from build123d import *

# Parameters (mm, degrees)
SKETCH1_W           = 80
SKETCH1_H           = 65
BOSS_EXTRUDE1_DEPTH = 10
SKETCH2_W           = 75
SKETCH2_H           = 60
CUT_EXTRUDE1_DEPTH  = 8
FILLET4_R           = 2
FILLET5_R           = 3
SKETCH3_W           = 80
SKETCH3_H           = 65
SKETCH3_W_2         = 77
SKETCH3_H_2         = 62
CUT_EXTRUDE2_DEPTH  = 1.5
FILLET7_R           = 4
SKETCH4_R           = 1.27
BOSS_EXTRUDE2_DEPTH = 3
SKETCH5_W           = 6
SKETCH5_H           = 3.5
CUT_EXTRUDE3_DEPTH  = 102.642756751
FILLET8_R           = 0.5
SKETCH8_W           = 69
SKETCH8_H           = 3
CUT_EXTRUDE4_DEPTH  = 1.5
SKETCH9_W           = 69
SKETCH9_H           = 3
CUT_EXTRUDE5_DEPTH  = 1.5


with BuildPart() as part:
    # Sketch1 → Boss-Extrude1 (new body)
    with BuildSketch(Plane(origin=(0, 0, 0), x_dir=(1, 0, 0), z_dir=(0, 1, 0))):
        with Locations((40, 32.5)):
            Rectangle(SKETCH1_W, SKETCH1_H)
    extrude(amount=BOSS_EXTRUDE1_DEPTH)

    # Sketch2 → Cut-Extrude1 (cut)
    with BuildSketch(Plane(origin=(0, 10, 0), x_dir=(1, 0, 0), z_dir=(0, 1, 0))):
        with Locations((40, 32.5)):
            Rectangle(SKETCH2_W, SKETCH2_H)
    extrude(amount=-CUT_EXTRUDE1_DEPTH, mode=Mode.SUBTRACT)

    # Fillet4
    fillet4_edges = [part.edges().sort_by_distance(p)[0] for p in [
        (40, 0, -65),
        (80, 0, -32.5),
        (40, 0, 0),
        (0, 0, -32.5),
    ]]
    fillet(fillet4_edges, radius=FILLET4_R)

    # Fillet5
    # the kernel refuses this fillet: 3 mm, written as the material it adds along each edge
    with BuildSketch(Plane(origin=(2.5, 10, -2.5), x_dir=(0, 0, -1), z_dir=(0, -1, 0)), Plane(origin=(77.5, 10, -62.5), x_dir=(0, 0, 1), z_dir=(0, -1, 0)), Plane(origin=(77.5, 10, -2.5), x_dir=(-1, 0, 0), z_dir=(0, -1, 0))) as fillet5_piece_1:
        with BuildLine():
            CenterArc((FILLET5_R, FILLET5_R), FILLET5_R, 180, 90)
            Line((0, FILLET5_R), (0, 0))
            Line((0, 0), (FILLET5_R, 0))
        make_face()
    extrude(amount=8)
    with BuildSketch(Plane(origin=(2.5, 10, -62.5), x_dir=(0, 0, 1), z_dir=(0, -1, 0))) as fillet5_piece_2:
        with BuildLine():
            CenterArc((FILLET5_R, -FILLET5_R), FILLET5_R, 90, 90)
            Line((0, -FILLET5_R), (0, 0))
            Line((0, 0), (FILLET5_R, 0))
        make_face()
    extrude(amount=8)
    # the kernel refuses this fillet: 3 mm, written as the material it takes off along each edge
    with BuildSketch(Plane(origin=(77, 0, -62), x_dir=(0, 0, -1), z_dir=(-1, 0, 0))) as fillet5_2_piece_1:
        with BuildLine():
            CenterArc((1, -2), 2, 0, 90)
            Line((3, -2), (3, 0))
            Line((3, 0), (1, 0))
        make_face()
    revolve(axis=Axis((77, 0, -62), (0, -1, 0)), revolution_arc=90, mode=Mode.SUBTRACT)
    with BuildSketch(Plane(origin=(77, 0, -3), x_dir=(1, 0, 0), z_dir=(0, 0, -1))) as fillet5_2_piece_2:
        with BuildLine():
            CenterArc((1, -2), 2, 0, 90)
            Line((3, -2), (3, 0))
            Line((3, 0), (1, 0))
        make_face()
    revolve(axis=Axis((77, 0, -3), (0, -1, 0)), revolution_arc=90, mode=Mode.SUBTRACT)
    with BuildSketch(Plane(origin=(3, 0, -62), x_dir=(-1, 0, 0), z_dir=(0, 0, 1))) as fillet5_2_piece_3:
        with BuildLine():
            CenterArc((1, -2), 2, 0, 90)
            Line((3, -2), (3, 0))
            Line((3, 0), (1, 0))
        make_face()
    revolve(axis=Axis((3, 0, -62), (0, -1, 0)), revolution_arc=90, mode=Mode.SUBTRACT)
    with BuildSketch(Plane(origin=(3, 0, -3), x_dir=(0, 0, 1), z_dir=(1, 0, 0))) as fillet5_2_piece_4:
        with BuildLine():
            CenterArc((1, -2), 2, 0, 90)
            Line((3, -2), (3, 0))
            Line((3, 0), (1, 0))
        make_face()
    revolve(axis=Axis((3, 0, -3), (0, -1, 0)), revolution_arc=90, mode=Mode.SUBTRACT)
    with BuildSketch(Plane(origin=(0, 0, -65), x_dir=(0, 0, 1), z_dir=(0, 1, 0)), Plane(origin=(0, 0, 0), x_dir=(1, 0, 0), z_dir=(0, 1, 0))) as fillet5_2_piece_5:
        with BuildLine():
            CenterArc((FILLET5_R, FILLET5_R), FILLET5_R, 180, 90)
            Line((0, FILLET5_R), (0, 0))
            Line((0, 0), (FILLET5_R, 0))
        make_face()
    extrude(amount=17.5, mode=Mode.SUBTRACT)
    with BuildSketch(Plane(origin=(80, 0, -65), x_dir=(0, 0, 1), z_dir=(0, 1, 0)), Plane(origin=(80, 0, 0), x_dir=(-1, 0, 0), z_dir=(0, 1, 0))) as fillet5_2_piece_6:
        with BuildLine():
            CenterArc((FILLET5_R, -FILLET5_R), FILLET5_R, 90, 90)
            Line((0, -FILLET5_R), (0, 0))
            Line((0, 0), (FILLET5_R, 0))
        make_face()
    extrude(amount=17.5, mode=Mode.SUBTRACT)

    # Sketch3 → Cut-Extrude2 (cut)
    with BuildSketch(Plane(origin=(0, 10, 0), x_dir=(1, 0, 0), z_dir=(0, 1, 0))):
        with Locations((40, 32.5)):
            Rectangle(SKETCH3_W, SKETCH3_H)
        with Locations((40, 32.5)):
            Rectangle(SKETCH3_W_2, SKETCH3_H_2, mode=Mode.SUBTRACT)
    extrude(amount=-CUT_EXTRUDE2_DEPTH, mode=Mode.SUBTRACT)

    # Fillet7
    fillet7_edges = [part.edges().sort_by_distance(p)[0] for p in [
        (78.5, 9.25, -63.5),
        (78.5, 9.25, -1.5),
        (1.5, 9.25, -1.5),
        (1.5, 9.25, -63.5),
    ]]
    fillet(fillet7_edges, radius=FILLET7_R)

    # Sketch4 → Boss-Extrude2 (add)
    with BuildSketch(Plane(origin=(0, 2, 0), x_dir=(1, 0, 0), z_dir=(0, 1, 0))):
        with Locations(Location((5.04, 8.04, 0), (0, 0, 270))):
            Circle(SKETCH4_R)
        with Locations(Location((5.04, 25.76, 0), (0, 0, 270))):
            Circle(SKETCH4_R)
        with Locations(Location((22.64, 34.64, 0), (0, 0, 270))):
            Circle(SKETCH4_R)
        with Locations(Location((22.64, 49.96, 0), (0, 0, 270))):
            Circle(SKETCH4_R)
        with Locations(Location((50.96, 8.04, 0), (0, 0, 270))):
            Circle(SKETCH4_R)
        with Locations(Location((50.96, 25.76, 0), (0, 0, 270))):
            Circle(SKETCH4_R)
        with Locations(Location((50.96, 34.64, 0), (0, 0, 270))):
            Circle(SKETCH4_R)
        with Locations(Location((50.96, 49.96, 0), (0, 0, 270))):
            Circle(SKETCH4_R)
    extrude(amount=BOSS_EXTRUDE2_DEPTH)

    # Sketch5 → Cut-Extrude3 (cut, through all)
    with BuildSketch(Plane(origin=(2.5, 0, 0), x_dir=(0, 0, -1), z_dir=(1, 0, 0))):
        with Locations((16.9, 6.25)):
            Rectangle(SKETCH5_W, SKETCH5_H)
    extrude(amount=-CUT_EXTRUDE3_DEPTH, mode=Mode.SUBTRACT)

    # Fillet8
    fillet8_edges = [part.edges().sort_by_distance(p)[0] for p in [
        (1.25, 4.5, -19.9),
        (1.25, 4.5, -13.9),
        (1.25, 8, -13.9),
        (1.25, 8, -19.9),
    ]]
    fillet(fillet8_edges, radius=FILLET8_R)

    # Sketch8 → Cut-Extrude4 (cut)
    with BuildSketch(Plane.XY.offset(-62.5)):
        with Locations((40, 6)):
            Rectangle(SKETCH8_W, SKETCH8_H)
    extrude(amount=-CUT_EXTRUDE4_DEPTH, mode=Mode.SUBTRACT)

    # Sketch9 → Cut-Extrude5 (cut)
    with BuildSketch(Plane(origin=(0, 0, -2.5), x_dir=(-1, 0, 0), z_dir=(0, 0, -1))):
        with Locations((-40, 6)):
            Rectangle(SKETCH9_W, SKETCH9_H)
    extrude(amount=-CUT_EXTRUDE5_DEPTH, mode=Mode.SUBTRACT)


solid = part.part
Verification items for the finished model (mm, model axes). A direction names the side the tool comes from. Give positions to 0.01 mm unless a question says otherwise; leave off trailing zeros. Loops run counter-clockwise (first coordinate to the right, second up) from the corner with the lowest first, then second, coordinate; pieces in that order, holes last.
1) Set-up check for faces 1 (the flat face through (40, 6, -64)), 2 (the cylindrical face through (77.297, 9.24, -62.359)), 3 (the flat face through (2.5, 6, -32)), 4 (the cylindrical face through (0.86, 5.2, -0.9)): record each of +Z, -Z, +X, -X, +Y, -Y from which the full face is reachable in a straight line by a thin tool's end or side.
2) Sectioned sample at A-A, the plane x = 33. Enter the section's corners in (y, z).
3) Draft check along X on faces 5 (the flat face through (80, 5, -32)), 6 (the flat face through (40, 3, -62.5)), 7 (the cylindrical face through (40.52, 0.6, -0.57)). Enter one of: pulls with the +X half, pulls with the -X half, needs draft (parallel to the pull), parting line crosses it, or undercut.
4) Thickness scan on line 1 along Z through (x, y) = (44, 8); line 2 along Z through (x, y) = (44, 5.5); line 3 along X through (y, z) = (3.5, -59). Record the ranges inside material, lowest first.
5) Sectioned sample at B-B, the plane z = -28. Enter the section's corners in (x, y), then the cut area to 3 significant figures.
6) Sectioned sample at C-C, the plane y = 6. Enter the section's corners in (x, z).
7) Depth check by flat-ended pin: pin 1 Ø1 at (x, z) = (35.5, -55) entering from +Y; pin 2 Ø0.8 at (x, y) = (47, 9) entering from +Z; pin 3 Ø1.3 at (x, z) = (51.5, -26.5) entering from +Y. Enter the tip coordinate at first touch or a pass-through.
Answers:
1. face 1: none
1. face 2: -Z, +X, +Y
1. face 3: +Y
1. face 4: +Z, -X, +Y, -Y
2. outline: (0, -63) arc R2 ccw to (2, -65) - (8.5, -65) - (8.5, -63.5) - (10, -63.5) - (10, -62.5) - (7.5, -62.5) - (7.5, -64) - (4.5, -64) - (4.5, -62.5) - (2, -62.5) - (2, -2.5) - (4.5, -2.5) - (4.5, -1) - (7.5, -1) - (7.5, -2.5) - (10, -2.5) - (10, -1.5) - (8.5, -1.5) - (8.5, 0) - (2, 0) arc R2 ccw to (0, -2) - close
3. face 5: pulls with the +X half
3. face 6: undercut
3. face 7: needs draft
4. line 1: z = -65 to -62.5, -2.5 to 0
4. line 2: z = -65 to -64, -1 to 0
4. line 3: x = 0 to 2.5, 77.5 to 80
5. outline: (0, 2) arc R2 ccw to (2, 0) - (78, 0) arc R2 ccw to (80, 2) - (80, 8.5) - (78.5, 8.5) - (78.5, 10) - (77.5, 10) - (77.5, 2) - (2.5, 2) - (2.5, 10) - (1.5, 10) - (1.5, 8.5) - (0, 8.5) - close
5. area: 194 mm2
6. outline: (0, -62) arc R3 ccw to (3, -65) - (77, -65) arc R3 ccw to (80, -62) - (80, -3) arc R3 ccw to (77, 0) - (3, 0) arc R3 ccw to (0, -3) - (0, -13.9) - (2.5, -13.9) - (2.5, -5.5) arc R3 cw to (5.5, -2.5) - (5.5, -1) - (74.5, -1) - (74.5, -2.5) arc R3 cw to (77.5, -5.5) - (77.5, -59.5) arc R3 cw to (74.5, -62.5) - (74.5, -64) - (5.5, -64) - (5.5, -62.5) arc R3 cw to (2.5, -59.5) - (2.5, -19.9) - (0, -19.9) - close
7. pin 1: stops at y = 2
7. pin 2: stops at z = -1.5
7. pin 3: stops at y = 5
